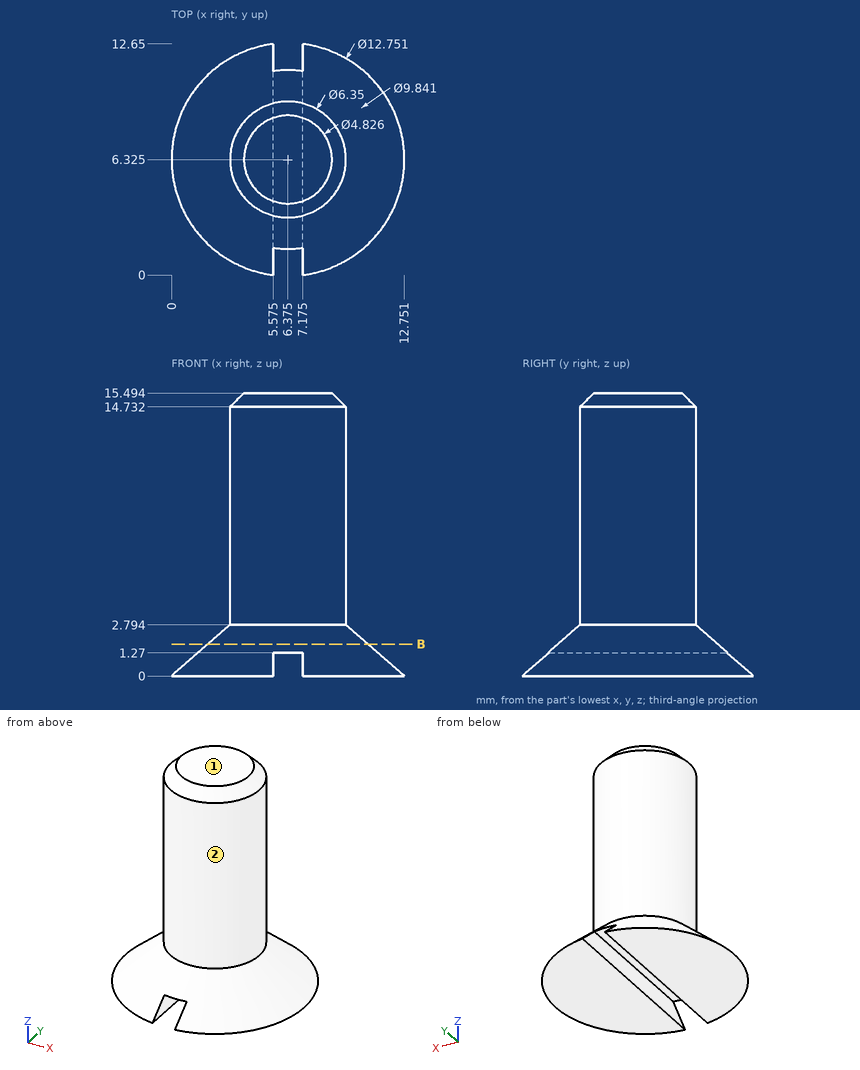
Design review of the part shown in the three views and the two pictorial views. Dimensions are in mm from the part's minimum x, y and z. A direction names the side the tool comes from. Round coordinates to 2 decimals unless told otherwise and drop trailing zeros. Write each loop counter-clockwise with the first axis right and the second up, starting at its lowest first coordinate (ties: lowest second). Pieces come first, ordered by that corner, then holes. Notation, with made-up numbers: M 1.5,20 L 24.5,20 A8 ccw 24.5,29 Z; hole C 43.25,6 d3. An arc over 180 degrees is marked long. One line per item, written item: value. Start each with the question number.
1. Take a section at B-B on z = 1.75. State the section outline as (x, y) points (1 decimal), then the cut area to 3 significant figures.
2. For the marked faces 1 and 2, list the 3-axis set-ups (+Z, -Z, +X, -X, +Y, -Y) from which the entire face can be reached by the end or side of a thin tool; tool diameter is ignored.
3. Clearance check with flat-ended pins moving along their axes: P1, Ø1, axis at y = 9.5, z = 0.5, coming from the -X side; P2, Ø1, axis at x = 9, z = 3, coming from the +Y side (1 decimal). State where each tip first meets the part, or that it passes through.
4. To check wall thickness, follow probe 1 along Z at (x, y) = (6.75, 8.25) (1 decimal); probe 2 along Y at (x, z) = (6.25, 4.75); probe 3 along X at (y, z) = (9, 9.25) (1 decimal). State the ranges of each line that lie inside material, in increasing order. Write a range as from..to.
Computed:
1. outline: C 6.4,6.3 d8.7
1. area: 60.0 mm²
2. face 1: +Z, +X, -X, +Y, -Y
2. face 2: +Z
3. P1: stops at x = 0.79
3. P2: stops at y = 8.8
4. probe 1: z = 1.3..15.5
4. probe 2: y = 3.15..9.5
4. probe 3: x = 4.7..8.1
